Study the drawing (mm; zero at the part's minimum x, y, z) and answer. A direction names the side the tool comes from. Give positions to 0.01 mm unless a question says otherwise; leave off trailing zeros. Write each loop counter-clockwise with the first axis right and the second up, starting at its lowest first coordinate (ties: lowest second). Pieces come first, ordered by that corner, then holes. Notation, with made-up numbers: (-19.75, 19.25) - (16.25, 19.25) arc R24 ccw to (16.25, 43.25) - close; hole circle Ø10 at (29.25, -4). An arc over 180 degrees is marked (long way). Return JSON: item names as keys, results as strings.
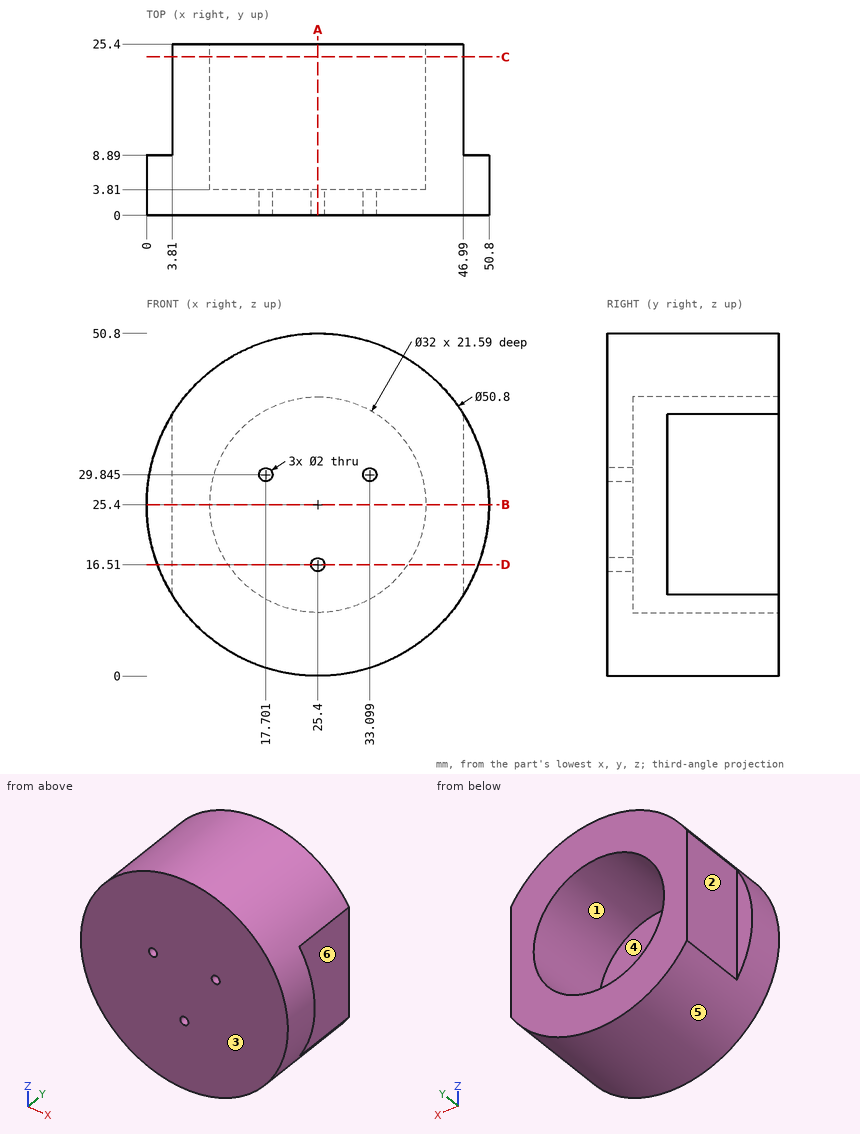
Item 1: The mould has two halves that part along X. Classify the marked faces 4, 5 and 6: +X half, -X half, draft (parallel to the pull), parting line (faces both ways), or undercut.
Answer below:
{"face 4": "undercut", "face 5": "parting line", "face 6": "+X half"}
Item 2: A cutting plane is placed at A-A on x = 25.4. Determine the outline of the cut face in (y, z), then the cut area to 3 significant figures.
Answer below:
{"outline": "(0, 0) - (25.4, 0) - (25.4, 9.4) - (3.81, 9.4) - (3.81, 15.51) - (0, 15.51) - close; (0, 17.51) - (3.81, 17.51) - (3.81, 41.4) - (25.4, 41.4) - (25.4, 50.8) - (0, 50.8) - close", "area": "592 mm²"}
Item 3: A cutting plane is placed at D-D on z = 16.51. Determine the outline of the cut face in (x, y), then the cut area to 3 significant figures.
Answer below:
{"outline": "(1.61, 0) - (24.4, 0) - (24.4, 3.81) - (12.1, 3.81) - (12.1, 25.4) - (3.81, 25.4) - (3.81, 8.89) - (1.61, 8.89) - close; (26.4, 0) - (49.19, 0) - (49.19, 8.89) - (46.99, 8.89) - (46.99, 25.4) - (38.7, 25.4) - (38.7, 3.81) - (26.4, 3.81) - close", "area": "554 mm²"}
Item 4: For the marked faces 1, 2 and 3, determine the directions among +Z, -Z, +X, -X, +Y, -Y from which every point of the face is accessible in a straight line to the end or side of a thin tool.
Answer below:
{"face 1": "+Y", "face 2": "+Z, -Z, -X, +Y", "face 3": "+Z, -Z, +X, -X, -Y"}
Item 5: A cutting plane is placed at B-B on z = 25.4. Determine the outline of the cut face in (x, y), then the cut area to 3 significant figures.
Answer below:
{"outline": "(0, 0) - (50.8, 0) - (50.8, 8.89) - (46.99, 8.89) - (46.99, 25.4) - (41.4, 25.4) - (41.4, 3.81) - (9.4, 3.81) - (9.4, 25.4) - (3.81, 25.4) - (3.81, 8.89) - (0, 8.89) - close", "area": "474 mm²"}
Item 6: A cutting plane is placed at C-C on y = 23.5. Determine the outline of the cut face in (x, z).
Answer below:
{"outline": "(3.81, 12.02) arc R25.4 ccw to (46.99, 12.02) - (46.99, 38.78) arc R25.4 ccw to (3.81, 38.78) - close; hole circle Ø32 at (25.4, 25.4)"}
Item 7: Flat-ended cylindrical pins translate along their axes: P1, Ø5, axis at x = 42.5, y = 7.5, coming from the +Z side; P2, Ø5, axis at y = 18, z = 31.5, coming from the -X side; P3, Ø8, axis at x = 26.5, z = 21, coming from the +Y side; P4, Ø3, axis at x = 17.7, z = 29.84, coming from the -Y side. Find the tip coordinate at first contact, or state that the pin passes through.
Answer below:
{"P1": "stops at z = 46.18", "P2": "stops at x = 3.81", "P3": "stops at y = 3.81", "P4": "stops at y = 0"}
Item 8: Consider L1, parallel to X at y = 22.5, z = 25 (3 decimals); L2, parallel to X at y = 12, z = 40 (1 decimal); L3, parallel to Z at x = 20, y = 6.75. Determine where each line is inside the solid, lowest interval first.
Answer below:
{"L1": "x = 3.81 to 9.405, 41.395 to 46.99", "L2": "x = 4.6 to 18.9, 31.9 to 46.2", "L3": "z = 0.58 to 10.34, 40.46 to 50.22"}
